Autodesk Inventor part; units mm, degrees
ref_plane "YZ Plane" through (0, 0, 0) normal (1, 0, 0) x (0, 1, 0)
ref_plane "XZ Plane" through (0, 0, 0) normal (0, 1, 0) x (-1, 0, 0)
ref_plane "XY Plane" through (0, 0, 0) normal (0, 0, 1) x (1, 0, 0)
sketch "Boceto1" plane through (0, 0, 0) normal (0, 0, 1) x (1, 0, 0)
  line L0 (-20, 20) -> (20, 20)
  line L1 (20, 20) -> (20, -20)
  line L2 (20, -20) -> (-20, -20)
  line L3 (-20, -20) -> (-20, 20)
  line L4 (-20, 20) -> (20, -20) construction
  line L5 (-18, 18) -> (18, 18)
  line L6 (18, 18) -> (18, -18)
  line L7 (18, -18) -> (-18, -18)
  line L8 (-18, -18) -> (-18, 18)
  line L9 (-18, 0) -> (-20, 0) construction
  line L10 (0, 18) -> (0, 20) construction
  line L11 (18, 0) -> (20, 0) construction
  line L12 (0, -18) -> (0, -20) construction
  point P0 (0, 0)
  point P1 (0, 0)
  dimension "d0" = 40
  dimension "d1" = 2
extrude "Extrusión1" add sketch "Boceto1" along normal blind 805
properties part number "C_358_40_2"
Input: part model. Units: mm. Frame: model coordinates. A direction names the side the tool comes from. Coordinates: 2 decimals unless noted, no trailing zeros. Loops run counter-clockwise (first coordinate to the right, second up) from the corner with the lowest first, then second, coordinate; pieces in that order, holes last.
Q1. Draft query along Y for faces 1 (the face through (0, 18, 397)), 2 (the face through (-2, -19, 805)), 3 (the face through (0, -18, 397)), 4 (the face through (0, 20, 397)). Return one class per face: +Y half, -Y half, draft (parallel to the pull), parting line (faces both ways), or undercut.
Q2. Cut plane A-A (x = -3.5). Output: boundary loops of the cut face in (y, z), then the cut area to 3 significant figures.
Q3. Material intervals for line 1 (Y direction, x = -12, z = 548), sorted ascending.
Q4. Set-up query: faces 5 (the face through (-2, -19, 0)), 6 (the face through (18, 0, 397)). Return all of +Z, -Z, +X, -X, +Y, -Y with unobstructed straight access to the full face (end or side cutting, diameter ignored); none if empty.
Q5. Cut plane C-C (z = 488). Output: boundary loops of the cut face in (x, y).
Working result:
1. face 1: undercut
1. face 2: draft
1. face 3: undercut
1. face 4: +Y half
2. outline: (-20, 0) - (-18, 0) - (-18, 805) - (-20, 805) - close; (18, 0) - (20, 0) - (20, 805) - (18, 805) - close
2. area: 3,220 mm2
3. line 1: y = -20 to -18, 18 to 20
4. face 5: -Z, +X, -X, +Y, -Y
4. face 6: +Z, -Z
5. outline: (-20, -20) - (20, -20) - (20, 20) - (-20, 20) - close; hole (-18, -18) - (18, -18) - (18, 18) - (-18, 18) - close
